```python
from build123d import *

# Parameters (mm, degrees)
F1_DEPTH  = 500
F2_W      = 273.5948168963
F2_H      = 203
F2_W_2    = 90
F2_H_2    = 80
F3_DEPTH  = 25
F2_R      = 7.5
F4_DEPTH  = 25
F5_R      = 25
F6_DEPTH  = 25
F8_DEPTH  = 15
F10_DEPTH = 15


with BuildPart() as f1:
    # F0 (on Top) → F1 (new body)
    with BuildSketch(Plane.XY):
        Polygon((123.0739113364, 227.9723018915), (-30.9260886636, 227.9723018915), (-35.8010886636, 212.9723018915), (108.0739113364, 212.9723018915), (108.0739113364, -157.0276981085), (-156.0510886636, -157.0276981085), (-160.9260886636, -172.0276981085), (123.0739113364, -172.0276981085), align=None)
        Polygon((-30.9260886636, 227.9723018915), (-46.6983942972, 227.9723018915), (-176.6983942972, -172.0276981085), (-160.9260886636, -172.0276981085), (-156.0510886636, -157.0276981085), (-35.8010886636, 212.9723018915), align=None)
    extrude(amount=F1_DEPTH)

    # F2 (on face) → F3 (cut)
    with BuildSketch(Plane(origin=(-109.2498744257, 35.5062091884, 0), x_dir=(-0.3090860723, -0.9510340687, 0), z_dir=(-0.9510340687, 0.3090860723, 0))):
        with Locations((7.4218059001, 378.5)):
            Rectangle(F2_W, F2_H)
        with Locations((16.6243974519, 87)):
            Rectangle(F2_W_2, F2_H_2)
    extrude(amount=-F3_DEPTH, mode=Mode.SUBTRACT)

    # F2 (on face) → F4 (cut)
    with BuildSketch(Plane(origin=(-109.2498744257, 35.5062091884, 0), x_dir=(-0.3090860723, -0.9510340687, 0), z_dir=(-0.9510340687, 0.3090860723, 0))):
        with Locations((-85.3756025481, 32.5)):
            Circle(F2_R)
    extrude(amount=-F4_DEPTH, mode=Mode.SUBTRACT)

    # F5 (on face) → F6 (cut)
    with BuildSketch(Plane.YZ.offset(123.0739113364)):
        with Locations((167.9723018915, 60)):
            Circle(F5_R)
    extrude(amount=-F6_DEPTH, mode=Mode.SUBTRACT)

    # F7 (on face) → F8 (join)
    with BuildSketch(Plane.XY.offset(500)):
        Polygon((123.0739113364, -172.0276981085), (123.0739113364, 227.9723018915), (-46.6983942972, 227.9723018915), (-176.6983942972, -172.0276981085), align=None)
    extrude(amount=F8_DEPTH)

    # F9 (on face) → F10 (join)
    with BuildSketch(Plane(origin=(0, 0, 0), x_dir=(1, 0, 0), z_dir=(0, 0, -1))):
        Polygon((-46.6983942972, -227.9723018915), (123.0739113364, -227.9723018915), (123.0739113364, 172.0276981085), (-176.6983942972, 172.0276981085), align=None)
    extrude(amount=F10_DEPTH)


solid = f1.part
```
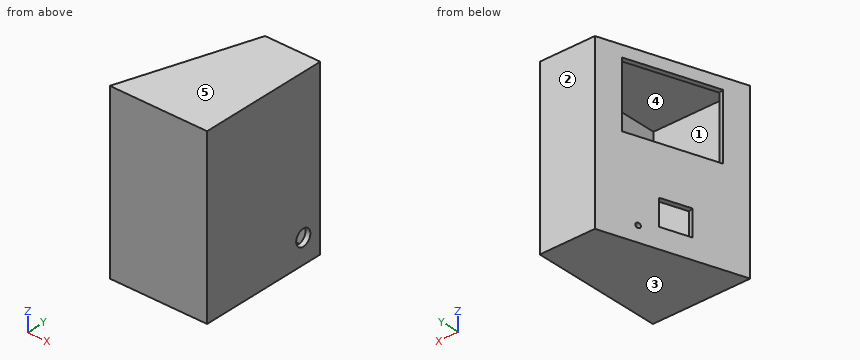
Build history of the part. All positions in model axes, mm. Face numbers are marked on the shaded views. A direction names the side the tool comes from. Round coordinates to 2 decimals unless told otherwise and drop trailing zeros. Write each loop counter-clockwise with the first axis right and the second up, starting at its lowest first coordinate (ties: lowest second). Pieces come first, ordered by that corner, then holes. Notation, with made-up numbers: (2, 23) - (7, 23) arc R20 ccw to (7, 37) - close; hole circle Ø1 at (-32.75, 53.5). An arc over 180 degrees is marked (long way). Answer as CSV lines item,"result".
Q1. Cut at C-C (z = 249.5). Write the cut outline in (x, y), and give its area (3 significant figures).
Report:
outline,"(-176.7, -172.03) - (123.07, -172.03) - (123.07, 227.97) - (-46.7, 227.97) - close; hole (-156.05, -157.03) - (108.07, -157.03) - (108.07, 212.97) - (-35.8, 212.97) - close"
area,"18,400 mm^2"
Q2. Drill centre lines: probe 1 along Y at (x, z) = (-29, 488.5); probe 2 along Z at (x, y) = (106, 57); probe 3 along X at (y, z) = (-91.5, 469.5). Where is each one in solid material? Low to high. Write a range as [from, to].
Report:
probe 1,"y = [-172.03, -157.03], [212.97, 227.97]"
probe 2,"z = [-15, 0], [500, 515]"
probe 3,"x = [108.07, 123.07]"
Q3. Cut at D-D (z = 413.5). Write the cut outline in (x, y).
Report:
outline,"(-176.7, -172.03) - (123.07, -172.03) - (123.07, 227.97) - (-46.7, 227.97) - (-69.26, 158.55) - (-55, 153.91) - (-35.8, 212.97) - (108.07, 212.97) - (108.07, -157.03) - (-156.05, -157.03) - (-139.56, -106.29) - (-153.83, -101.65) - close"
Q4. Pull direction Y, two halves, no side cores. Call the marked faces 1, 2 and 3: +Y half, -Y half, draft (parallel to the pull), parting line (faces both ways), or undercut.
Report:
face 1,"undercut"
face 2,"+Y half"
face 3,"draft"
Q5. Cut at B-B (x = 65). Write the cut outline in (y, z).
Report:
outline,"(-172.03, -15) - (227.97, -15) - (227.97, 515) - (-172.03, 515) - close; hole (-157.03, 0) - (212.97, 0) - (212.97, 500) - (-157.03, 500) - close"
Q6. Cut at A-A (z = 60). Write the cut outline in (x, y).
Report:
outline,"(-176.7, -172.03) - (123.07, -172.03) - (123.07, 142.97) - (108.07, 142.97) - (108.07, -157.03) - (-156.05, -157.03) - (-114.03, -27.74) - (-128.3, -23.1) - close; (-100.48, 62.49) - (-86.21, 57.86) - (-35.8, 212.97) - (108.07, 212.97) - (108.07, 192.97) - (123.07, 192.97) - (123.07, 227.97) - (-46.7, 227.97) - close"
Q7. Tool access for the marked faces 4 and 5: list every direction of +Z, -Z, +X, -X, +Y, -Y with a clear straight run to the whole face (end or side of a thin tool).
Report:
face 4,"none"
face 5,"+Z, +X, -X, +Y, -Y"
Q8. Drop flat-ended pins along their axis: pin 1 (10 mm diameter, centred on y = 45, z = 310.5, fed in from -X); pin 2 (1 mm diameter, centred on y = 176.5, z = 260, fed in from -X). Give the stop position or say it passes through.
Report:
pin 1,"stops at x = 108.07"
pin 2,"stops at x = -63.59"
